For this review, take the finished solid that the model builds, in its own axes (mm). A direction names the side the tool comes from. Round coordinates to 2 decimals unless told otherwise and drop trailing zeros. Loops run counter-clockwise (first coordinate to the right, second up) from the corner with the lowest first, then second, coordinate; pieces in that order, holes last.
1. Consider section B-B on x = 25.5. State the section outline as (y, z) points.
2. Consider section C-C on z = 41.5. State the section outline as (x, y) points, then the cut area to 3 significant figures.
3. Consider section A-A on y = 15. State the section outline as (x, z) points.
4. Tool access review of faces 5 (the flat face through (20, 15, 32)), 6 (the flat face through (26, 4, 32)), 7 (the cylindrical face through (0.43, 29.55, 30.42)): name each direction out of +Z, -Z, +X, -X, +Y, -Y from which nothing blocks a thin tool from reaching the whole face with its end or side.
5. To check wall thickness, follow line 1 along X through (y, z) = (15, 5.5); line 2 along Z through (x, y) = (22, 12.5); line 3 along X through (y, z) = (13.25, 42). State the ranges of each line that lie inside material, in increasing order.
6. Consider section D-D on x = 4.5. State the section outline as (y, z) points, then the cut area to 3 significant figures.
7. Clearance check with flat-ended pins moving along their axes: pin 1 Ø6 at (x, y) = (10.5, 16) entering from +Z; pin 2 Ø11 at (y, z) = (18.5, 24) entering from +X. State where each tip first meets the part, or that it passes through.
8. Draft analysis for pull direction Z (two halves, no side actions). For faces 1 (the flat face through (26, 15, 13.5)), 2 (the cylindrical face through (29.55, 0.43, 30.42)), 3 (the flat face through (21, 15, 60)), 4 (the flat face through (21, 15, 32)), state which applies: released by +Z, released by -Z, zero draft, split by the parting line, or undercut.
from build123d import *

# Parameters (mm, degrees)
BOX_W           = 30
BOX_H           = 30
BOX_DEPTH       = 60
SKETCH_W        = 18
SKETCH_H        = 27
POCKET_DEPTH    = 56
SKETCH001_W     = 22
SKETCH001_H     = 36
POCKET001_DEPTH = 9
SKETCH003_R     = 3.5
POCKET002_DEPTH = 13.5
SKETCH004_W     = 1.5
SKETCH004_H     = 3.5
POCKET003_DEPTH = 1
SKETCH005_W     = 3
SKETCH005_H     = 1.5
POCKET004_DEPTH = 1
FILLET_R        = 1.5
FILLET001_R     = 0.8


with BuildPart() as part:
    # Box → Box (new body)
    with BuildSketch(Plane.XY):
        with Locations((15, 15)):
            Rectangle(BOX_W, BOX_H)
    extrude(amount=BOX_DEPTH)

    # Sketch (on Face6 of BaseFeature) → Pocket (cut)
    with BuildSketch(Plane.XY.offset(60)):
        with Locations((11, 15)):
            Rectangle(SKETCH_W, SKETCH_H)
    extrude(amount=-POCKET_DEPTH, mode=Mode.SUBTRACT)

    # Sketch001 (on Face6 of Pocket) → Pocket001 (cut)
    with BuildSketch(Plane.YZ.offset(30)):
        with Locations((15, 32)):
            Rectangle(SKETCH001_W, SKETCH001_H)
    extrude(amount=-POCKET001_DEPTH, mode=Mode.SUBTRACT)

    # Sketch003 (on Face5 of Pocket001) → Pocket002 (cut)
    with BuildSketch(Plane(origin=(0, 0, 0), x_dir=(1, 0, 0), z_dir=(0, 0, -1))):
        with Locations((25.5, -15)):
            Circle(SKETCH003_R)
    extrude(amount=-POCKET002_DEPTH, mode=Mode.SUBTRACT)

    # Sketch004 (on Face17 of Pocket002) → Pocket003 (cut)
    with BuildSketch(Plane(origin=(0, 0, 13.5), x_dir=(1, 0, 0), z_dir=(0, 0, -1))):
        with Locations((23.75, -15)):
            Rectangle(SKETCH004_W, SKETCH004_H)
    extrude(amount=-POCKET003_DEPTH, mode=Mode.SUBTRACT)

    # Sketch005 (on Face18 of Pocket003) → Pocket004 (cut)
    with BuildSketch(Plane.YZ.offset(21)):
        with Locations((15, 47.25)):
            Rectangle(SKETCH005_W, SKETCH005_H)
    extrude(amount=-POCKET004_DEPTH, mode=Mode.SUBTRACT)

    # Fillet
    fillet_edges = [part.edges().sort_by_distance(p)[0] for p in [
        (30, 0, 30),
        (30, 30, 30),
        (0, 0, 30),
        (0, 30, 30),
    ]]
    fillet(fillet_edges, radius=FILLET_R)

    # Fillet001
    fillet001_edges = [part.edges().sort_by_distance(p)[0] for p in [
        (25.5, 26, 50),
        (25.5, 26, 14),
        (25.5, 4, 14),
        (25.5, 4, 50),
    ]]
    fillet(fillet001_edges, radius=FILLET001_R)


solid = part.part
Resolved:
1. outline: (0, 0) - (11.5, 0) - (11.5, 13.5) - (18.5, 13.5) - (18.5, 0) - (30, 0) - (30, 60) - (0, 60) - close; hole (4, 14.8) arc R0.8 ccw to (4.8, 14) - (25.2, 14) arc R0.8 ccw to (26, 14.8) - (26, 49.2) arc R0.8 ccw to (25.2, 50) - (4.8, 50) arc R0.8 ccw to (4, 49.2) - close
2. outline: (0, 1.5) arc R1.5 ccw to (1.5, 0) - (28.5, 0) arc R1.5 ccw to (30, 1.5) - (30, 4) - (21, 4) - (21, 26) - (30, 26) - (30, 28.5) arc R1.5 ccw to (28.5, 30) - (1.5, 30) arc R1.5 ccw to (0, 28.5) - close; hole (2, 1.5) - (20, 1.5) - (20, 28.5) - (2, 28.5) - close
2. area: 214 mm2
3. outline: (0, 0) - (22, 0) - (22, 13.5) - (23, 13.5) - (23, 14) - (21, 14) - (21, 46.5) - (20, 46.5) - (20, 4) - (2, 4) - (2, 60) - (0, 60) - close; (20, 48) - (21, 48) - (21, 50) - (30, 50) - (30, 60) - (20, 60) - close; (24.5, 13.5) - (29, 13.5) - (29, 0) - (30, 0) - (30, 14) - (24.5, 14) - close
4. face 5: +Z
4. face 6: +X
4. face 7: +Z, -Z, -X, +Y
5. line 1: x = 0 to 2, 20 to 22, 29 to 30
5. line 2: z = 0 to 14, 50 to 60
5. line 3: x = 0 to 2, 20 to 21
6. outline: (0, 0) - (30, 0) - (30, 60) - (28.5, 60) - (28.5, 4) - (1.5, 4) - (1.5, 60) - (0, 60) - close
6. area: 288 mm2
7. pin 1: stops at z = 4
7. pin 2: stops at x = 21
8. face 1: released by -Z
8. face 2: zero draft
8. face 3: released by +Z
8. face 4: undercut
